Input: part model. Units: mm. Frame: model coordinates. A direction names the side the tool comes from. Coordinates: 2 decimals unless noted, no trailing zeros. Loops run counter-clockwise (first coordinate to the right, second up) from the corner with the lowest first, then second, coordinate; pieces in that order, holes last. Notation, with made-up numbers: (12.5, -17.5) - (60.5, -17.5) arc R11 cw to (60.5, 0.5) - close; hole circle Ø9 at (-3.5, 0.25). An arc over 180 degrees is marked (long way). Use a Markdown table: item, result. Add a question column.
1. Ray query, L1, parallel to Z at x = 4, y = -8.5; L2, parallel to Y at x = -0.5, z = -49.5; L3, parallel to X at y = 0.75, z = -28. Return the intervals inside material, ascending. Write a range as [from, to].
2. Access query for faces 4 (the face through (3.421, 1, -43)), 5 (the face through (2, -23.5, -69)), 6 (the face through (4, 1, -74.382)), 7 (the face through (3, -14, -62.883)). Directions: +Z, -Z, +X, -X, +Y, -Y. A direction counts if a zero-diameter tool reaches every point of the face in a straight line with its end or side. Return the directions, or none.
3. Contact query for flat-ended pins moving along their axis: P1, Ø0.9, axis at x = -8.5, z = -83.5, coming from the -Y side; P2, Ø1, axis at x = -0.5, z = -38.5, coming from the -Y side; P3, Ø8, axis at y = -12.5, z = -65.5, coming from the -X side. Output: stop coordinate, or through.
4. Section query B-B on y = -19.25. Return the cut outline in (x, z).
5. Draft query along Y for faces 1 (the face through (-8, -15, -27)), 2 (the face through (0.92, -23.8, -68.6)), 3 (the face through (3.421, -19, -69)). Return one class per face: released by +Y, released by -Y, zero draft, split by the parting line, or undercut.
6. Section query A-A on x = 1.5. State how many separate pieces and enclosed holes the cut face has, then the cut area to 3 significant figures.
7. Section query D-D on z = -56. Return the cut outline in (x, y), then the cut area to 3 significant figures.
Autodesk Inventor part; units mm, degrees
ref_plane "YZ Plane" through (0, 0, 0) normal (1, 0, 0) x (0, 1, 0)
ref_plane "XZ Plane" through (0, 0, 0) normal (0, 1, 0) x (-1, 0, 0)
ref_plane "XY Plane" through (0, 0, 0) normal (0, 0, 1) x (1, 0, 0)
sketch "Sketch7" plane through (0, 0, 0) normal (0, 1, 0) x (-1, 0, 0)
  line L0 (13.5789, -22.6329) -> (-3.4211, -22.6329)
  line L1 (-3.4211, -22.6329) -> (-3.4211, -87.6329)
  line L2 (-3.4211, -87.6329) -> (13.5789, -87.6329)
  line L3 (13.5789, -87.6329) -> (13.5789, -22.6329)
  point P0 (0, 0)
  dimension "d16" = 65
  dimension "d17" = 17
extrude "Extrusion4" add sketch "Sketch7" along normal blind 2
fillet "Fillet1" radius 1 4 edges at (3.4211, 1, -22.6329) (-13.5789, 1, -22.6329) (3.4211, 1, -87.6329) (-13.5789, 1, -87.6329)
sketch "Sketch15" plane through (0, 0, 0) normal (0, -1, 0) x (1, 0, 0)
  line L0 (-13.5789, -86.6329) -> (-13.5789, -23.6329)
  line L1 (-13.5789, -55.1329) -> (3.4211, -55.1329)
  line L2 (3.4211, -23.6329) -> (3.4211, -86.6329)
  line L3 (-13.5789, -55.1329) -> (-13.5789, -68.6329)
  circle A0 centre (-13.5789, -68.6329) radius 4
  circle A1 centre (-13.5789, -41.6329) radius 4
  point P0 (0, 0)
  dimension "d46" = 13.5
  dimension "d47" = 8
extrude "Extrusion8" cut sketch "Sketch15" against normal blind 5
sketch "Sketch16" plane through (0, 0, 0) normal (0, -1, 0) x (1, 0, 0)
  arc A0 (-13.5789, -72.6329) -> (-13.5789, -64.6329) centre (-13.5789, -68.6329) ccw
  line L0 (-13.5789, -68.6329) -> (-7.7855, -83.2432)
  line L1 (-13.5789, -68.6329) -> (2.1381, -68.6329) construction
  circle A1 centre (-7.7855, -83.2432) radius 1.5
  line L2 (-13.5789, -64.6329) -> (-13.5789, -45.6329) construction
  line L3 (-13.5789, -55.1329) -> (3.4211, -55.1329) construction
  line L4 (3.4211, -23.6329) -> (3.4211, -86.6329) construction
  line L5 (-13.5789, -41.6329) -> (-7.7855, -27.0227)
  circle A2 centre (-7.7855, -27.0227) radius 1.5
  circle A3 centre (-7.7855, -83.2432) radius 2
  circle A4 centre (-7.7855, -27.0227) radius 2
  point P0 (0, 0)
  dimension "d50" = 15.717
  dimension "d51" = 68.37
  dimension "d52" = 3
  dimension "d55" = 4
  dimension "d56" = 4
extrude "Extrusion9" add sketch "Sketch16" along normal blind 15 contours A1 | A2
sketch "Sketch17" plane through (0, 2, 0) normal (0, 1, 0) x (1, 0, 0)
  line L0 (-12.5789, 22.6329) -> (2.4211, 22.6329) construction
  line L1 (0, 22.6329) -> (0, 87.6329) construction
  line L2 (2.4211, 87.6329) -> (-12.5789, 87.6329) construction
  arc A0 (-13.5789, 64.6329) -> (-13.5789, 72.6329) centre (-13.5789, 68.6329) ccw construction
  line L3 (-13.5789, 68.6329) -> (3.4211, 68.6329) construction
  line L4 (3.4211, 23.6329) -> (3.4211, 86.6329) construction
  line L5 (-9.5789, 62.8384) -> (-9.5789, 74.4274) construction
  point P0 (0, 0)
  point P1 (-9.5789, 68.6329)
  dimension "d57" = 11.589
sketch "Sketch25" plane through (0, 2, 0) normal (0, 1, 0) x (1, 0, 0)
  line L0 (3.4211, 23.6329) -> (3.4211, 86.6329)
  arc A0 (-13.5789, 64.6329) -> (-13.5789, 72.6329) centre (-13.5789, 68.6329) ccw
  point P0 (0, 0)
sketch "Sketch27" plane through (3.4211, 0, -86.6329) normal (1, 0, 0) x (0, 0, -1)
  line L0 (-63, 2) -> (0, 2)
  line L1 (-23.7493, 0) -> (-12.2507, 0)
  line L2 (-12.2507, 0) -> (-12.2507, 2)
  line L3 (-12.2507, 2) -> (-23.7493, 2)
  line L4 (-23.7493, 2) -> (-23.7493, 0)
  point P0 (-86.6329, 0)
extrude "Extrusion16" add sketch "Sketch27" along normal blind 1.5
sketch "Sketch28" plane through (0, 0, 0) normal (0, -1, 0) x (1, 0, 0)
  line L0 (4.9211, -74.3823) -> (3.4211, -74.3823)
  line L1 (3.4211, -74.3823) -> (3.4211, -62.8836)
  line L2 (3.4211, -62.8836) -> (4.9211, -62.8836)
  line L3 (4.9211, -62.8836) -> (4.9211, -74.3823)
  point P0 (0, 0)
extrude "Extrusion17" add sketch "Sketch28" along normal blind 24
sketch "Sketch29" plane through (4.9211, 0, -86.6329) normal (1, 0, 0) x (0, 0, -1)
  line L0 (-22, 2) -> (-14, 2) construction
  line L1 (-18, 2) -> (-18, -24) construction
  line L2 (-23.7493, -24) -> (-12.2507, -24) construction
  circle A0 centre (-20.1722, -20.5985) radius 0.5
  circle A1 centre (-15.8278, -20.5985) radius 0.5
  point P0 (-86.6329, 0)
  dimension "d97" = 1
hole "Hole4" at (4.9211, -20.5985, -66.4608) at (4.9211, -20.5985, -70.8051) direction (-1, 0, 0) diameter 1 end through all
sketch "Sketch31" plane through (4.9211, 2, -74.3823) normal (0, 0, -1) x (-1, 0, 0)
  point P0 (4.9211, -2)
sketch "Sketch35" plane through (4.9211, 2, -74.3823) normal (0, 0, -1) x (-1, 0, 0)
  point P0 (4.9211, -2)
sketch "Sketch36" plane through (4.9211, 2, -74.3823) normal (0, 0, -1) x (-1, 0, 0)
  line L0 (1.5, -26) -> (1.5, -14)
  line L1 (1.5, -2) -> (1.5, -26)
  line L2 (1.5, -14) -> (4.0015, -16.5015)
  line L3 (1.5, -14) -> (5.0376, -14) construction
  line L4 (4.0015, -16.5015) -> (1.5, -16.5015)
  point P0 (4.9211, -2)
  dimension "d111" = 12
  dimension "d112" = 45
extrude "Extrusion21" add sketch "Sketch36" against normal blind 11.499
sketch "Sketch38" plane through (4.9211, 2, -74.3823) normal (0, 0, -1) x (-1, 0, 0)
  line L0 (4.0015, -16.5015) -> (4.0015, -26)
  line L1 (4.0015, -26) -> (1.5, -26)
  line L2 (4.0015, -16.5015) -> (1.5, -16.5015)
  line L3 (1.5, -16.5015) -> (4.0015, -16.5015)
  line L4 (1.5, -16.5015) -> (1.5, -26)
  point P0 (4.9211, -2)
sketch "Sketch39" plane through (3.4211, 2, -62.8836) normal (0, 0, 1) x (1, 0, 0)
  line L0 (-2.5015, -16.5015) -> (-2.5015, -26)
  line L1 (-2.5015, -26) -> (0, -26)
  line L2 (0, -26) -> (1.5, -26)
  line L3 (-2.5015, -16.5015) -> (0, -16.5015)
  line L4 (-2.5015, -16.5015) -> (0, -16.5015)
  line L5 (0, -16.5015) -> (0, -26)
  line L6 (0, -16.5015) -> (0, -26)
  point P0 (-3.4211, -2)
extrude "Extrusion22" add sketch "Sketch38" against normal blind 1
extrude "Extrusion23" add sketch "Sketch39" against normal blind 1
sketch "Sketch40" plane through (0, -24, 0) normal (0, -1, 0) x (1, 0, 0)
  line L0 (0.9196, -63.8836) -> (0.9196, -73.3823)
  line L1 (0.9196, -73.3823) -> (3.4211, -73.3823)
  line L2 (3.4211, -74.3823) -> (3.4211, -62.8836)
  line L3 (3.4211, -73.3823) -> (3.4211, -63.8836)
  line L4 (3.4211, -63.8836) -> (0.9196, -63.8836)
  line L5 (3.4211, -63.8836) -> (0.9196, -63.8836)
  point P0 (0, 0)
extrude "Extrusion24" add sketch "Sketch40" against normal blind 0.5
sketch "Sketch41" plane through (3.4211, -14.5015, -73.3823) normal (-1, 0, 0) x (0, 0, 1)
  point P0 (73.3823, 14.5015)
properties part number "Latch"
Resolved:
| question | item | result |
|---|---|---|
| 1 | L1 | [-74.38, -62.88] |
| 1 | L2 | [0, 2] |
| 1 | L3 | [-13.58, 3.42] |
| 2 | face 4 | +Z, +X, +Y, -Y |
| 2 | face 5 | -X |
| 2 | face 6 | -Z, +X, +Y, -Y |
| 2 | face 7 | +Z, +X, -X, -Y |
| 3 | P1 | y = -15 |
| 3 | P2 | y = 0 |
| 3 | P3 | x = 0.92 |
| 4 | outline | (0.92, -74.38) - (4.92, -74.38) - (4.92, -62.88) - (0.92, -62.88) - (0.92, -63.88) - (3.42, -63.88) - (3.42, -73.38) - (0.92, -73.38) - close |
| 5 | face 1 | released by -Y |
| 5 | face 2 | zero draft |
| 5 | face 3 | undercut |
| 6 | separate pieces | 2 |
| 6 | enclosed holes | 1 |
| 6 | area | 160 mm² |
| 7 | outline | (-13.58, 0) - (3.42, 0) - (3.42, 2) - (-13.58, 2) - close |
| 7 | area | 34.0 mm² |
